from build123d import *

# Parameters (mm, degrees)
SKETCH1_R       = 3.175
EXTRUDE1_DEPTH  = 25.4
SKETCH2_R       = 4.953
EXTRUDE2_DEPTH  = 2.54
CHAMFER1_SIZE   = 0.508
SKETCH3_R       = 1.3890625
EXTRUDE3_DEPTH  = 5.953
LPATTERN1_COUNT = 6
LPATTERN1_PITCH = 6.35
CHAMFER2_SIZE   = 0.3175


with BuildPart() as part:
    # Sketch1 → Extrude1 (new body, symmetric)
    with BuildSketch(Plane.XY):
        Circle(SKETCH1_R)
    extrude(amount=EXTRUDE1_DEPTH, both=True)

    # Sketch2 → Extrude2 (add)
    with BuildSketch(Plane.XY.offset(25.4)):
        Circle(SKETCH2_R)
    extrude(amount=EXTRUDE2_DEPTH)

    # Chamfer1
    chamfer1_edges = [part.edges().sort_by_distance(p)[0] for p in [
        (-4.953, 0, 27.94),
    ]]
    chamfer(chamfer1_edges, length=CHAMFER1_SIZE)

    # Sketch3 → Extrude3 (cut, symmetric)
    with BuildSketch(Plane(origin=(0, 0, 0), x_dir=(0, 0, -1), z_dir=(1, 0, 0))):
        with Locations((19.05, 0)):
            Circle(SKETCH3_R)
    extrude3 = extrude(amount=EXTRUDE3_DEPTH, both=True, mode=Mode.SUBTRACT)

    # LPattern1: Extrude3 ×6
    with Locations(*[(0, 0, i * LPATTERN1_PITCH) for i in range(1, LPATTERN1_COUNT)]):
        add(extrude3, mode=Mode.SUBTRACT)

    # Chamfer2
    chamfer2_edges = [part.edges().sort_by_distance(p)[0] for p in [
        (-3.175, 0, -25.4),
    ]]
    chamfer(chamfer2_edges, length=CHAMFER2_SIZE)


solid = part.part
The listing builds one solid part. Answer for the finished solid, in the listing's coordinates (mm). Give positions to 0.01 mm unless a question says otherwise; leave off trailing zeros. Write each loop counter-clockwise with the first axis right and the second up, starting at its lowest first coordinate (ties: lowest second). Pieces come first, ordered by that corner, then holes. Notation, with made-up numbers: (45.25, 7.25) - (97.25, 7.25) arc R27 cw to (97.25, 34.25) - close; hole circle Ø3 at (80, 26). An arc over 180 degrees is marked (long way). Use a Markdown table: item, result.
1. Find the intervals of material crossed by probe 1 along Y at (x, z) = (0.75, -6.35); probe 2 along Y at (x, z) = (1, -11.5); probe 3 along Z at (x, y) = (3.75, -2), in increasing order. Write a range as from..to.
Values follow:
| item | result |
|---|---|
| probe 1 | y = -3.09..-1.39, 1.39..3.09 |
| probe 2 | y = -3.01..-0.7, 0.7..3.01 |
| probe 3 | z = 25.4..27.94 |
2. Section C-C on z = 6 is taken. Write down the section's boundary in (x, y) (3 decimals).
Values follow:
| item | result |
|---|---|
| outline | (-2.876, -1.344) arc R3.175 ccw to (2.876, -1.344) - close; (-2.876, 1.344) - (2.876, 1.344) arc R3.175 ccw to start |
3. Section A-A on x = 0 is taken. Count the separate pieces of the cut face and the enclosed holes in it, plus the area to 3 significant figures.
Values follow:
| item | result |
|---|---|
| separate pieces | 1 |
| enclosed holes | 6 |
| area | 311 mm² |
4. Section D-D on z = 20.5 is taken. Write down the section's boundary in (x, y) (3 decimals), plus the area to 3 significant figures.
Values follow:
| item | result |
|---|---|
| outline | circle Ø6.35 at (0, 0) |
| area | 31.7 mm² |
5. For a pull along Z with two mould halves and no side action, classify faces 1 (the cylindrical face through (0.043, -1.356, 6.651)), 2 (the flat face through (3.2, -1, 25.4)), 3 (the cylindrical face through (-2.52, -1.93, 0.51)) as released by +Z, released by -Z, zero draft, split by the parting line, or undercut.
Values follow:
| item | result |
|---|---|
| face 1 | undercut |
| face 2 | released by -Z |
| face 3 | zero draft |
6. Each of these flat-tipped pins is pushed along its axis until it touches: P1, Ø3.5, axis at y = 0, z = 0, coming from the -X side (3 decimals); P2, Ø3, axis at y = -3, z = -10.5, coming from the -X side; P3, Ø2.5, axis at y = 0, z = -12.7, coming from the +X side; P4, Ø3.5, axis at y = 0, z = 12.7, coming from the +X side (3 decimals). Where does it stop, or does it pass through?
Values follow:
| item | result |
|---|---|
| P1 | stops at x = -3.175 |
| P2 | stops at x = -2.8 |
| P3 | passes through |
| P4 | stops at x = 3.175 |
